Verification items for the finished model (mm, model axes). A direction names the side the tool comes from. Coordinates: 2 decimals unless noted, no trailing zeros. Order: outer loops, then holes, each group sorted by start corner. A loop starts at its lowest first (then second) coordinate and runs counter-clockwise, first axis right, second up. Notation, with made-up numbers: (14.25, 45) - (42.25, 45) arc R20 cw to (42.25, 61) - close; hole circle Ø4 at (81, 29.5). An arc over 180 degrees is marked (long way). Answer as CSV lines item,"result". Start each with the question number.
1. Section check A-A (z = 0.5). Record the cut outline in (x, y), and give its area (3 significant figures).
2. Section check C-C (y = 1.9). Record the cut outline in (x, z), and give its area (3 significant figures).
3. Mould release check, pull along Z, two halves, no side actions. Record for faces 3 (the flat face through (0, 1, -3.25)), 4 (the flat face through (0, 3, 0)), 5 (the flat face through (0, 1, -2.75)): pulls with the +Z half, pulls with the -Z half, needs draft (parallel to the pull), parting line crosses it, or undercut.
4. Section check B-B (y = 1.15). Record the cut outline in (x, z), and give its area (3 significant figures).
5. Material ranges on L1, parallel to Z at x = 0.25, y = 0.5; L2, parallel to Y at x = 0.75, z = -2.25, recorded low to high. Write a range as [from, to].
6. Set-up check for faces 1 (the flat face through (0, 1, 2.75)), 2 (the flat face through (3.25, 1.5, 0)): record each of +Z, -Z, +X, -X, +Y, -Y from which the full face is reachable in a straight line by a thin tool's end or side.
7. Section check D-D (x = -2.25). Record the cut outline in (y, z), and give its area (3 significant figures).
Autodesk Inventor part; units mm, degrees
ref_plane "YZ Plane" through (0, 0, 0) normal (1, 0, 0) x (0, 1, 0)
ref_plane "XZ Plane" through (0, 0, 0) normal (0, 1, 0) x (-1, 0, 0)
ref_plane "XY Plane" through (0, 0, 0) normal (0, 0, 1) x (1, 0, 0)
sketch "Sketch2" plane through (0, 0, 0) normal (0, 1, 0) x (-1, 0, 0)
  line L0 (-2.75, -2.75) -> (2.75, -2.75)
  line L1 (2.75, -2.75) -> (2.75, 2.75)
  line L2 (2.75, 2.75) -> (-2.75, 2.75)
  line L3 (-2.75, 2.75) -> (-2.75, -2.75)
  line L4 (-2.75, -2.75) -> (2.75, 2.75) construction
  line L5 (2.75, -2.75) -> (-2.75, 2.75) construction
  line L6 (3.25, 3.25) -> (-3.25, 3.25)
  line L7 (-3.25, 3.25) -> (-3.25, -3.25)
  line L8 (-3.25, -3.25) -> (3.25, -3.25)
  line L9 (3.25, -3.25) -> (3.25, 3.25)
  line L10 (3.25, 3.25) -> (-3.25, -3.25) construction
  line L11 (-3.25, 3.25) -> (3.25, -3.25) construction
  point P0 (0, 0)
  point P1 (3.25, 0)
  point P2 (-3.25, 0)
  point P3 (3.25, 0)
  point P4 (-3.25, 0)
  point P5 (3.25, 0)
  point P6 (2.75, 0)
  point P7 (-2.75, 0)
  dimension "d2" = 5.5
  dimension "d3" = 5.5
  dimension "d6" = 6.5
  dimension "d7" = 6.5
extrude "Extrusion1" add sketch "Sketch2" along normal blind 2
sketch "Sketch4" plane through (0, 2, 0) normal (0, 1, 0) x (1, 0, 0)
  line L0 (-3.25, 3.25) -> (-3.25, -3.25)
  line L1 (3.25, -3.25) -> (3.25, 3.25)
  line L2 (-3.25, -3.25) -> (3.25, -3.25)
  line L3 (3.25, -3.25) -> (3.25, 3.25)
  line L4 (3.25, 3.25) -> (-3.25, 3.25)
  line L5 (-3.25, 3.25) -> (-3.25, -3.25)
  point P0 (0, 0)
  dimension "d10" = 6.5
extrude "Extrusion2" add sketch "Sketch4" along normal blind 1
sketch "Sketch5" plane through (0, 0, 0) normal (0, -1, 0) x (1, 0, 0)
  line L0 (-3.25, -3.25) -> (-3.25, 3.25)
  line L1 (3.25, 3.25) -> (3.25, -3.25)
  point P0 (0, 0)
  point P1 (-3.25, 0)
  point P2 (3.25, 0)
sketch "Sketch6" plane through (2.75, 0, -2.75) normal (-1, 0, 0) x (0, 0, 1)
  line L0 (1.55, 0.4) -> (3.95, 0.4)
  line L1 (3.95, 0.4) -> (3.95, 1.6)
  line L2 (3.95, 1.6) -> (1.55, 1.6)
  line L3 (1.55, 1.6) -> (1.55, 0.4)
  line L4 (1.55, 0.4) -> (3.95, 1.6) construction
  line L5 (3.95, 0.4) -> (1.55, 1.6) construction
  line L6 (0, 2) -> (5.5, 2)
  point P0 (2.75, 0)
  point P1 (2.75, 1)
  dimension "d13" = 2.4
  dimension "d14" = 1.2
  dimension "d15" = 1
extrude "Extrusion3" cut sketch "Sketch6" against normal blind 0.5 draft -30
sketch "Sketch7" plane through (-2.75, 0, 2.75) normal (1, 0, 0) x (0, 0, -1)
  line L0 (1.55, 0.4) -> (3.95, 0.4)
  line L1 (3.95, 0.4) -> (3.95, 1.6)
  line L2 (3.95, 1.6) -> (1.55, 1.6)
  line L3 (1.55, 1.6) -> (1.55, 0.4)
  line L4 (1.55, 0.4) -> (3.95, 1.6) construction
  line L5 (3.95, 0.4) -> (1.55, 1.6) construction
  line L6 (0, 2) -> (5.5, 2)
  point P0 (2.75, 0)
  point P1 (2.75, 1)
  dimension "d18" = 2.4
  dimension "d19" = 1.2
  dimension "d20" = 1
extrude "Extrusion4" cut sketch "Sketch7" against normal blind 0.5 draft -30
properties part number "snapfit_lid_v07"
Evaluation:
1,outline,"(-3.25, 0) - (-2.75, 0) - (-2.75, 0.4) - (-3.25, 0.69) - close; (-3.25, 1.31) - (-2.75, 1.6) - (-2.75, 2) - (2.75, 2) - (2.75, 1.6) - (3.25, 1.31) - (3.25, 3) - (-3.25, 3) - close; (2.75, 0) - (3.25, 0) - (3.25, 0.69) - (2.75, 0.4) - close"
1,area,"7.59 mm²"
2,outline,"(-3.25, -3.25) - (3.25, -3.25) - (3.25, 3.25) - (-3.25, 3.25) - close; hole (-2.75, -2.75) - (2.75, -2.75) - (2.75, 2.75) - (-2.75, 2.75) - close"
2,area,"12.0 mm²"
3,face 3,"pulls with the -Z half"
3,face 4,"needs draft"
3,face 5,"undercut"
4,outline,"(-3.25, -3.25) - (3.25, -3.25) - (3.25, -0.91) - (2.75, -1.2) - (2.75, -2.75) - (-2.75, -2.75) - (-2.75, -1.2) - (-3.25, -0.91) - close; (-3.25, 0.91) - (-2.75, 1.2) - (-2.75, 2.75) - (2.75, 2.75) - (2.75, 1.2) - (3.25, 0.91) - (3.25, 3.25) - (-3.25, 3.25) - close"
4,area,"9.89 mm²"
5,L1,"z = [-3.25, -2.75], [2.75, 3.25]"
5,L2,"y = [2, 3]"
6,face 1,"-Y"
6,face 2,"+Z, -Z, +X, +Y, -Y"
7,outline,"(0, -3.25) - (3, -3.25) - (3, 3.25) - (0, 3.25) - (0, 2.75) - (2, 2.75) - (2, -2.75) - (0, -2.75) - close"
7,area,"8.50 mm²"
